Check sheet for the drawn part. Datum: minimum x, y, z corner. Units: mm. Round coordinates to 2 decimals unless told otherwise and drop trailing zeros. Write each loop counter-clockwise with the first axis right and the second up, starting at its lowest first coordinate (ties: lowest second). Pieces come first, ordered by that corner, then holes. Notation, with made-up numbers: M 7.5,-21.75 L 32.5,-21.75 A14 cw 32.5,-13.75 Z; hole C 55,16 d2. An arc over 180 degrees is marked long. Use a Markdown table: item, result.
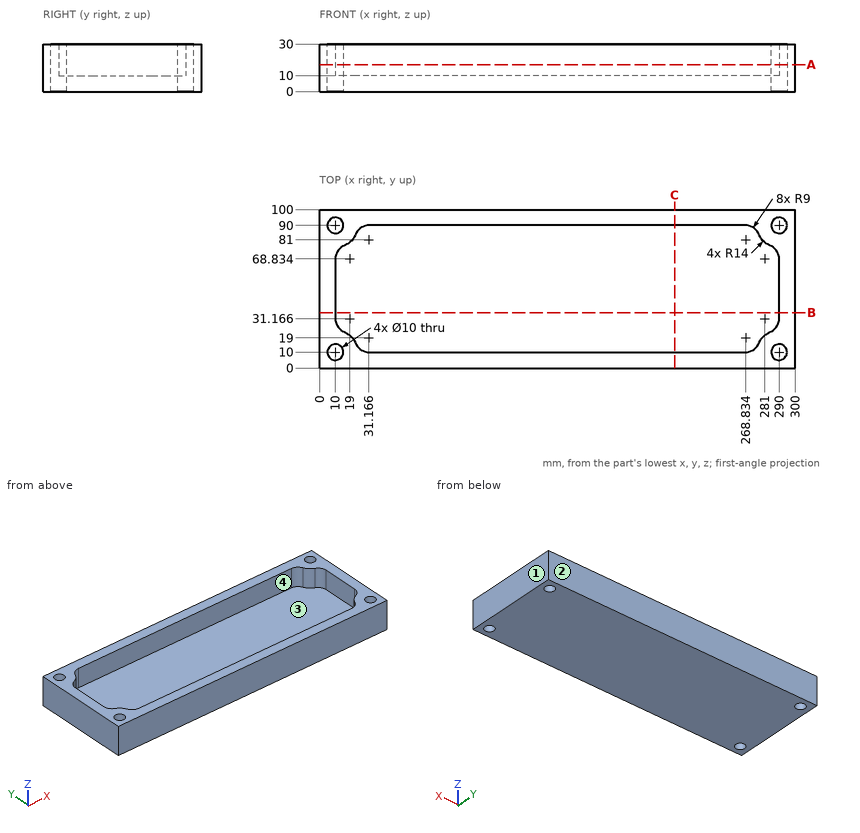
Item 1: Go/stop test with flat-tipped pins: pin 1 (8 mm diameter, centred on x = 10, y = 10, fed in from -Z); pin 2 (5 mm diameter, centred on x = 140, y = 36.5, fed in from +Z). Record where each tip stops, or that it passes through.
Outcome:
| item | result |
|---|---|
| pin 1 | passes through |
| pin 2 | stops at z = 10 |
Item 2: Cross-section at C-C, the plane x = 224. Record the cut outline in (y, z).
Outcome:
| item | result |
|---|---|
| outline | M 0,0 L 100,0 L 100,30 L 90,30 L 90,10 L 10,10 L 10,30 L 0,30 Z |
Item 3: Material ranges on line 1 along Y through (x, z) = (290, 7); line 2 along X through (y, z) = (64.5, 26.75); line 3 along X through (y, z) = (15.5, 24.75), recorded low to high. Write a range as from..to.
Outcome:
| item | result |
|---|---|
| line 1 | y = 0..5, 15..85, 95..100 |
| line 2 | x = 0..10, 290..300 |
| line 3 | x = 0..22.87, 277.13..300 |
Item 4: Mould release check, pull along Y, two halves, no side actions. Record for the marked faces 1, 2, 3 and 4: +Y half, -Y half, draft (parallel to the pull), parting line (faces both ways), or undercut.
Outcome:
| item | result |
|---|---|
| face 1 | draft |
| face 2 | +Y half |
| face 3 | undercut |
| face 4 | undercut |
Item 5: Cross-section at B-B, the plane y = 35. Record the cut outline in (x, z), and give its area (3 significant figures).
Outcome:
| item | result |
|---|---|
| outline | M 0,0 L 300,0 L 300,30 L 290,30 L 290,10 L 10,10 L 10,30 L 0,30 Z |
| area | 3,400 mm2 |
Item 6: Cross-section at A-A, the plane z = 17. Record the cut outline in (x, y), and give its area (3 significant figures).
Outcome:
| item | result |
|---|---|
| outline | M 0,0 L 300,0 L 300,100 L 0,100 Z; hole C 10,10 d10; hole C 10,90 d10; hole M 10,31.17 A9 ccw 15.48,22.88 A14 cw 22.88,15.48 A9 ccw 31.17,10 L 268.83,10 A9 ccw 277.12,15.48 A14 cw 284.52,22.88 A9 ccw 290,31.17 L 290,68.83 A9 ccw 284.52,77.12 A14 cw 277.12,84.52 A9 ccw 268.83,90 L 31.17,90 A9 ccw 22.88,84.52 A14 cw 15.48,77.12 A9 ccw 10,68.83 Z; hole C 290,10 d10; hole C 290,90 d10 |
| area | 7,970 mm2 |
